The figure shows three views and two pictorial views of one solid part (mm, origin at its lowest corner). Answer the questions. Give positions to 0.01 mm unless a question says otherwise; leave off trailing zeros. Order: outer loops, then holes, each group sorted by start corner. A loop starts at its lowest first (then second) coordinate and runs counter-clockwise, first axis right, second up. Notation, with made-up numbers: (36.25, 43.25) - (49.25, 43.25) arc R12 ccw to (49.25, 63.25) - close; hole circle Ø6 at (-26.5, -22). An arc over 180 degrees is marked (long way). Answer as a JSON object with one key per item and string values. Group by question number.
Q1. A cutting plane is placed at C-C, the plane y = 7.5. Give the vertices of the cut face in (x, z), and give its area (3 significant figures).
Q2. A cutting plane is placed at B-B, the plane z = 1.65. Give the vertices of the cut face in (x, y).
Q3. Consider line 1 (X direction, y = 67.5, z = 1.1); line 2 (Y direction, x = 15.5, z = 0.7); line 3 (X direction, y = 67, z = 1.5). Determine where each line is inside the solid, lowest interval first.
Q4. Given pin 1 (1 mm diameter, centred on x = 2, z = 1, fed in from +Y); pin 2 (5 mm diameter, centred on x = 15.5, y = 67.5, fed in from -Z); pin 3 (0.6 mm diameter, centred on y = 72, z = 0.5, fed in from -X), each flat-ended and moving along its own axis, determine where each tip first touches the part or whether it passes through.
Q5. A cutting plane is placed at A-A, the plane x = 75.5. Give the vertices of the cut face in (y, z).
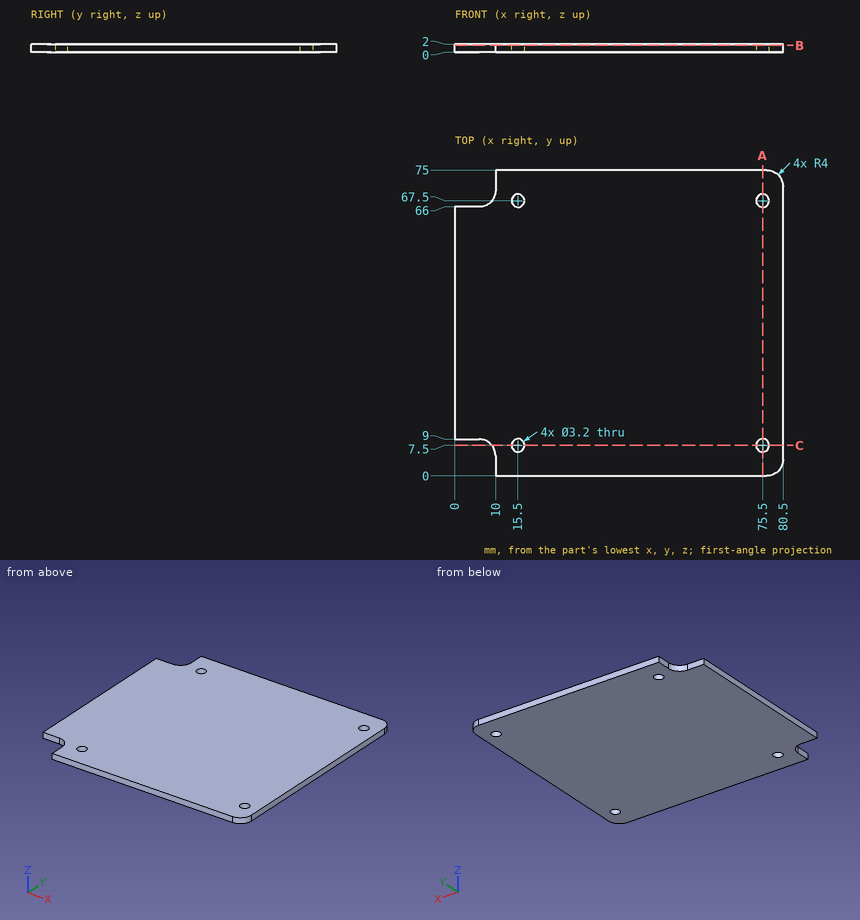
Reply:
{
 "1": {"outline": "(9.12, 0) - (13.9, 0) - (13.9, 2) - (9.12, 2) - close; (17.1, 0) - (73.9, 0) - (73.9, 2) - (17.1, 2) - close; (77.1, 0) - (80.5, 0) - (80.5, 2) - (77.1, 2) - close", "area": "130 mm^2"},
 "2": {"outline": "(0, 9) - (6, 9) arc R4 cw to (10, 5) - (10, 0) - (76.5, 0) arc R4 ccw to (80.5, 4) - (80.5, 71) arc R4 ccw to (76.5, 75) - (10, 75) - (10, 70) arc R4 cw to (6, 66) - (0, 66) - close; hole circle Ø3.2 at (15.5, 7.5); hole circle Ø3.2 at (15.5, 67.5); hole circle Ø3.2 at (75.5, 7.5); hole circle Ø3.2 at (75.5, 67.5)"},
 "3": {"line 1": "x = 9.12 to 13.9, 17.1 to 73.9, 77.1 to 80.5", "line 2": "y = 0 to 5.9, 9.1 to 65.9, 69.1 to 75", "line 3": "x = 8.65 to 13.98, 17.02 to 73.98, 77.02 to 80.5"},
 "4": {"pin 1": "stops at y = 66", "pin 2": "stops at z = 0", "pin 3": "stops at x = 10"},
 "5": {"outline": "(0, 0) - (5.9, 0) - (5.9, 2) - (0, 2) - close; (9.1, 0) - (65.9, 0) - (65.9, 2) - (9.1, 2) - close; (69.1, 0) - (75, 0) - (75, 2) - (69.1, 2) - close"}
}
